Geometry: final body of the model. Coordinates: model frame, mm. Give positions to 0.01 mm unless a question says otherwise; leave off trailing zeros. Order: outer loops, then holes, each group sorted by start corner. A loop starts at its lowest first (then second) coordinate and runs counter-clockwise, first axis right, second up. Notation, with made-up numbers: (28, 9) - (84, 9) arc R28 cw to (84, 31) - close; hole circle Ø7 at (41.25, -26). An arc over 180 degrees is marked (long way). Write item = value, one per line. Start each with the question number.
from build123d import *

# Parameters (mm, degrees)
SKETCH1_R           = 3.5
SKETCH1_W           = 90
SKETCH1_H           = 30
SKETCH1_W_2         = 7
SKETCH1_H_2         = 3.9
BOSS_EXTRUDE1_DEPTH = 4
SKETCH4_W           = 6
SKETCH4_H           = 2
BOSS_EXTRUDE2_DEPTH = 4
CHAMFER1_SIZE       = 2
CUT_EXTRUDE1_REACH  = 52.426
SKETCH5_R           = 1.1
SKETCH6_R           = 2
CUT_EXTRUDE2_DEPTH  = 2


with BuildPart() as part:
    # Sketch1 → Boss-Extrude1 (new body)
    with BuildSketch(Plane(origin=(0, 0, 0), x_dir=(1, 0, 0), z_dir=(0, 1, 0))):
        with Locations((0, 18.9)):
            Circle(SKETCH1_R)
        Rectangle(SKETCH1_W, SKETCH1_H)
        with Locations((0, 16.95)):
            Rectangle(SKETCH1_W_2, SKETCH1_H_2)
    extrude(amount=BOSS_EXTRUDE1_DEPTH)

    # Sketch4 → Boss-Extrude2 (add)
    with BuildSketch(Plane.XY.offset(15)):
        with Locations((-20, 1)):
            Rectangle(SKETCH4_W, SKETCH4_H)
        with Locations((20, 1)):
            Rectangle(SKETCH4_W, SKETCH4_H)
    extrude(amount=BOSS_EXTRUDE2_DEPTH)

    # Chamfer1
    chamfer1_edges = [part.edges().sort_by_distance(p)[0] for p in [
        (20, 0, 19),
        (-20, 0, 19),
    ]]
    chamfer(chamfer1_edges, length=CHAMFER1_SIZE - 0.0001)  # a hair under: the kernel refuses the full size

    # Sketch5 → Cut-Extrude1 (cut, up to next)
    with BuildSketch(Plane(origin=(0, 4, 0), x_dir=(1, 0, 0), z_dir=(0, 1, 0)), mode=Mode.PRIVATE) as cut_extrude1_sk1:
        with Locations(Location((0, 18.9, 0), (0, 0, 270))):
            Circle(SKETCH5_R)
    cut_extrude1_tool1 = extrude(cut_extrude1_sk1.sketch, amount=-CUT_EXTRUDE1_REACH, mode=Mode.PRIVATE) & part.part
    add(cut_extrude1_tool1.solids().sort_by_distance((0, 4, -18.9))[0], mode=Mode.SUBTRACT)

    # Sketch6 → Cut-Extrude2 (cut)
    with BuildSketch(Plane(origin=(0, 4, 0), x_dir=(1, 0, 0), z_dir=(0, 1, 0))):
        with Locations(Location((0, 18.9, 0), (0, 0, 270))):
            Circle(SKETCH6_R)
    extrude(amount=-CUT_EXTRUDE2_DEPTH, mode=Mode.SUBTRACT)


solid = part.part
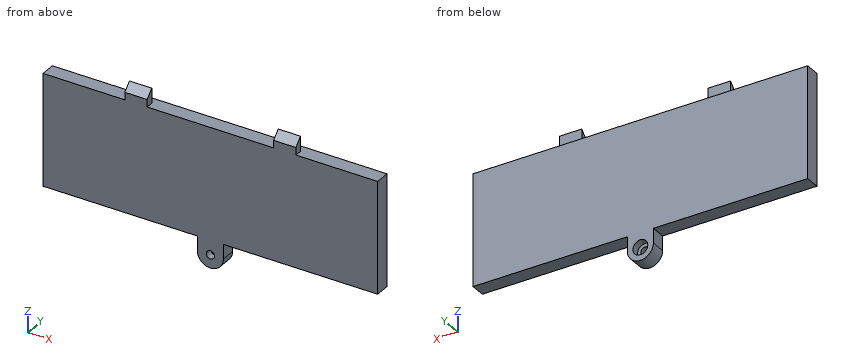
Q1. Contact query for flat-ended pins moving along their axis: pin 1 (1.6 mm diameter, centred on y = 1, z = 16, fed in from +X); pin 2 (1.2 mm diameter, centred on x = -21, z = 17.5, fed in from +Y); pin 3 (1.9 mm diameter, centred on y = 1.5, z = -17.5, fed in from -X). Output: stop coordinate, or through.
Q2. Section A-A, the plane x = 0. Return the cut outline in (y, z).
Q3. Material intervals for line 1 along X through (y, z) = (0.65, -18.9); line 2 along X through (y, z) = (2.3, -19); line 3 along Z through (x, y) = (-37, 1.15), sorted ascending. Write a range as from..to.
Q4. Section B-B, the plane y = 0.7. Return the cut outline in (x, z).
Q5. Section C-C, the plane x = -26.5. Return the cut outline in (y, z), then the cut area to 3 significant figures.
The answers:
q1.pin_1 = 23
q1.pin_2 = 2
q1.pin_3 = -3.5
q2.outline = (0, -22.4) - (4, -22.4) - (4, -20.9) - (2, -20.9) - (2, -20) - (0, -20) - close; (0, -17.8) - (2, -17.8) - (2, -16.9) - (4, -16.9) - (4, 15) - (0, 15) - close
q3.line_1 = -3.5..-1.1, 1.1..3.5
q3.line_2 = -3.5..-2, 2..3.5
q3.line_3 = -15..15
q4.outline = (-45, -15) - (-3.5, -15) - (-3.5, -18.9) arc R3.5 ccw to (3.5, -18.9) - (3.5, -15) - (45, -15) - (45, 15) - (23, 15) - (23, 17.7) - (17, 17.7) - (17, 15) - (-17, 15) - (-17, 17.7) - (-23, 17.7) - (-23, 15) - (-45, 15) - close; hole circle Ø2.2 at (0, -18.9)
q5.outline = (0, -15) - (4, -15) - (4, 15) - (0, 15) - close
q5.area = 120 mm²
